```python
from build123d import *

# Parameters (mm, degrees)
SKETCH3_W               = 31
SKETCH3_H               = 31
BOSS_EXTRUDE2_DEPTH     = 4
SKETCH4_W               = 25
SKETCH4_H               = 25
CUT_EXTRUDE1_DEPTH      = 3
SKETCH5_W               = 23
SKETCH5_H               = 23
CUT_EXTRUDE2_DEPTH      = 5
SKETCH9_R               = 1.5
CUT_EXTRUDE3_DEPTH      = 10
MIRROR3_COPY_1_SKETCH_R = 1.5
MIRROR3_COPY_1_DEPTH    = 10
CUT_EXTRUDE4_DEPTH      = 37.84087404


with BuildPart() as part:
    # Sketch3 → Boss-Extrude2 (new body)
    with BuildSketch(Plane.XY):
        Rectangle(SKETCH3_W, SKETCH3_H)
    extrude(amount=BOSS_EXTRUDE2_DEPTH)

    # Sketch4 → Cut-Extrude1 (cut)
    with BuildSketch(Plane.XY.offset(4)):
        Rectangle(SKETCH4_W, SKETCH4_H)
    extrude(amount=-CUT_EXTRUDE1_DEPTH, mode=Mode.SUBTRACT)

    # Sketch5 → Cut-Extrude2 (cut)
    with BuildSketch(Plane.XY.offset(1)):
        Rectangle(SKETCH5_W, SKETCH5_H)
    extrude(amount=-CUT_EXTRUDE2_DEPTH, mode=Mode.SUBTRACT)

    # Sweep1: sweep along a curve in space
    with BuildLine() as sweep1_path:
        Line((-15.5, -15.5, 4), (15.5, -15.5, 4))
    # Sketch6 → Sweep1 (sweep)
    with BuildSketch(Plane.ZY.offset(15.5)):
        Polygon((4, -15.5), (4, -19.5), (0, -15.5), align=None)
    sweep(path=sweep1_path.line)

    # Sweep2: sweep along a curve in space
    with BuildLine() as sweep2_path:
        Line((15.5, 15.5, 0), (-15.5, 15.5, 0))
    # Sketch8 → Sweep2 (sweep)
    with BuildSketch(Plane.ZY.offset(15.5)):
        Polygon((0, 15.5), (4, 19.43634716), (4, 15.5), align=None)
    sweep(path=sweep2_path.line)

    # Sketch9 → Cut-Extrude3 (cut)
    with BuildSketch(Plane(origin=(0, 0, 0), x_dir=(-1, 0, 0), z_dir=(0, 0, -1))):
        with Locations((-12.5, 15.5)):
            Circle(SKETCH9_R)
    cut_extrude3 = extrude(amount=-CUT_EXTRUDE3_DEPTH, mode=Mode.SUBTRACT)

    # Mirror1: Cut-Extrude3 across plane
    add(cut_extrude3.mirror(Plane(origin=(0, 0, 0), x_dir=(0, 0, 1), z_dir=(1, 0, 0))), mode=Mode.SUBTRACT)

    # Mirror3: Cut-Extrude3 across plane
    add(cut_extrude3.mirror(Plane.ZX), mode=Mode.SUBTRACT)

    # Mirror3 copy 1 sketch → Mirror3 copy 1 (cut)
    with BuildSketch(Plane(origin=(0, 0, 0), x_dir=(1, 0, 0), z_dir=(0, 0, -1))):
        with Locations((-12.5, 15.5)):
            Circle(MIRROR3_COPY_1_SKETCH_R)
    extrude(amount=-MIRROR3_COPY_1_DEPTH, mode=Mode.SUBTRACT)

    # Sketch10 → Cut-Extrude4 (cut, through all)
    with BuildSketch(Plane.ZY.offset(15.5)):
        Polygon((0, -15.5), (1.5, -17), (1.5, -13.5), (0, -13.5), align=None)
        Polygon((1.524255803, 17), (0, 15.5), (0, 13.5), (1.524255803, 13.5), align=None)
    extrude(amount=-CUT_EXTRUDE4_DEPTH, mode=Mode.SUBTRACT)


solid = part.part
```
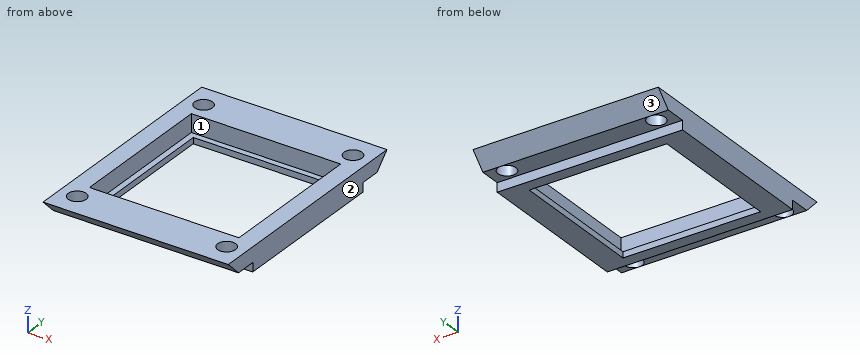
Input: part model. Units: mm. Frame: model coordinates. Face numbers are marked on the shaded views. Give positions to 0.01 mm unless a question says otherwise; leave off trailing zeros. Order: outer loops, then holes, each group sorted by start corner. A loop starts at its lowest first (then second) coordinate and runs counter-clockwise, first axis right, second up. Notation, with made-up numbers: (44, -32.75) - (55, -32.75) arc R17 ccw to (55, -21.75) - close; hole circle Ø4 at (-13.5, 74.25). An arc over 180 degrees is marked (long way). One line per item, written item: value.
1. Draft query along Y for the marked faces 1, 2 and 3. Return one class per face: released by +Y, released by -Y, zero draft, split by the parting line, or undercut.
Determined:
face 1: undercut
face 2: zero draft
face 3: released by +Y
2. Cut plane A-A, the plane y = -5. Output: boundary loops of the cut face in (x, z), and give its area (3 significant figures).
Determined:
outline: (-15.5, 0) - (-11.5, 0) - (-11.5, 1) - (-12.5, 1) - (-12.5, 4) - (-15.5, 4) - close; (11.5, 0) - (15.5, 0) - (15.5, 4) - (12.5, 4) - (12.5, 1) - (11.5, 1) - close
area: 26.0 mm2
3. Pin query (flat end, axial travel): pin 1 Ø1.8 at (x, y) = (4, -14.5) entering from -Z; pin 2 Ø1.2 at (x, z) = (-7.5, 0.5) entering from -Y; pin 3 Ø0.9 at (x, z) = (5, 2) entering from -Y. Return the tip coordinate at first contact, or that it passes through.
Determined:
pin 1: z = 1.5
pin 2: y = -13.5
pin 3: y = -17.95
4. Cut plane B-B, the plane x = 3.5. Output: boundary loops of the cut face in (y, z).
Determined:
outline: (-19.5, 4) - (-17, 1.5) - (-13.5, 1.5) - (-13.5, 0) - (-11.5, 0) - (-11.5, 1) - (-12.5, 1) - (-12.5, 4) - close; (11.5, 0) - (13.5, 0) - (13.5, 1.52) - (17, 1.52) - (19.44, 4) - (12.5, 4) - (12.5, 1) - (11.5, 1) - close
5. Line query: probe 1 along X at (y, z) = (15.5, 3.3); probe 2 along Y at (x, z) = (3, 0.35); probe 3 along X at (y, z) = (0.5, 0.4). Output: solid intervals per line, ascending.
Determined:
probe 1: -15.5 to -14, -11 to 11, 14 to 15.5
probe 2: -13.5 to -11.5, 11.5 to 13.5
probe 3: -15.5 to -11.5, 11.5 to 15.5
6. Cut plane D-D, the plane z = 3.25. Output: boundary loops of the cut face in (x, y), and give its area (3 significant figures).
Determined:
outline: (-15.5, -18.75) - (15.5, -18.75) - (15.5, 18.7) - (-15.5, 18.7) - close; hole circle Ø3 at (-12.5, -15.5); hole circle Ø3 at (-12.5, 15.5); hole (-12.5, -12.5) - (12.5, -12.5) - (12.5, 12.5) - (-12.5, 12.5) - close; hole circle Ø3 at (12.5, -15.5); hole circle Ø3 at (12.5, 15.5)
area: 508 mm2
7. Cut plane C-C, the plane y = 15.5. Output: boundary loops of the cut face in (x, z).
Determined:
outline: (-15.5, 1.52) - (-14, 1.52) - (-14, 4) - (-15.5, 4) - close; (-11, 1.52) - (11, 1.52) - (11, 4) - (-11, 4) - close; (14, 1.52) - (15.5, 1.52) - (15.5, 4) - (14, 4) - close
